Source: CAD feature listing. Evaluate the final solid. Frame: model axes, mm. A direction names the side the tool comes from. Round coordinates to 2 decimals unless told otherwise and drop trailing zeros. Write each loop counter-clockwise with the first axis right and the second up, starting at its lowest first coordinate (ties: lowest second). Pieces come first, ordered by that corner, then holes.
from build123d import *

# Parameters (mm, degrees)
SKETCH1_W                      = 140
SKETCH1_H                      = 44
BASE_FLANGE1_DEPTH             = 1.9
EDGE_FLANGE1_DEPTH             = 140
EDGE_FLANGE1_2_DEPTH           = 140
EDGE_FLANGE2_STRIP_CUT_DEPTH   = 140
EDGE_FLANGE2_STRIP_CUT_2_DEPTH = 140
EDGE_FLANGE2_DEPTH             = 140
EDGE_FLANGE2_BEND_DEPTH        = 140
SKETCH40_R                     = 1
CUT_EXTRUDE1_DEPTH             = 5


# Read off the part's stored shape, not the designer's step: Edge-Flange1
# Sheet-metal steps are written as plain solids
with BuildPart() as part:
    # Sketch1 → Base-Flange1 (new body)
    with BuildSketch(Plane.XY):
        with Locations((70, 22)):
            Rectangle(SKETCH1_W, SKETCH1_H)
    extrude(amount=-BASE_FLANGE1_DEPTH)

    # Edge-Flange1 outline → Edge-Flange1 (cut)
    with BuildSketch(Plane.YZ):
        with BuildLine():
            ThreePointArc((41.266511693, 0), (42.824680557, -0.454164807), (43.894804276, -1.674407041))
            Line((43.894804276, -1.674407041), (44, -1.9))
            Line((44, -1.9), (44, 0))
            Line((44, 0), (41.266511693, 0))
        make_face()
        with BuildLine():
            ThreePointArc((0.105195724, -1.674407041), (1.175319443, -0.454164807), (2.733488307, 0))
            Line((2.733488307, 0), (0, 0))
            Line((0, 0), (0, -1.9))
            Line((0, -1.9), (0.105195724, -1.674407041))
        make_face()
    extrude(amount=EDGE_FLANGE1_DEPTH, mode=Mode.SUBTRACT)

    # Edge-Flange1 2 outline → Edge-Flange1 2 (add)
    with BuildSketch(Plane.YZ):
        with BuildLine():
            Line((44.259494142, -2.456486983), (44, -1.9))
            Line((44, -1.9), (41.266511693, -1.9))
            ThreePointArc((41.266511693, -1.9), (41.803811302, -2.056608554), (42.17281948, -2.477381738))
            Line((42.17281948, -2.477381738), (42.537509347, -3.259461681))
            Line((42.537509347, -3.259461681), (44.259494142, -2.456486983))
        make_face()
        with BuildLine():
            ThreePointArc((1.82718052, -2.477381738), (2.196188698, -2.056608554), (2.733488307, -1.9))
            Line((2.733488307, -1.9), (0, -1.9))
            Line((0, -1.9), (-0.259494142, -2.456486983))
            Line((-0.259494142, -2.456486983), (1.462490653, -3.259461681))
            Line((1.462490653, -3.259461681), (1.82718052, -2.477381738))
        make_face()
    extrude(amount=EDGE_FLANGE1_2_DEPTH)

    # Edge-Flange2 strip (across the edge) → Edge-Flange2 strip cut (cut)
    with BuildSketch(Plane(origin=(140, 44.259494142, -2.456486983), x_dir=(0, 0, 1), z_dir=(-1, 0, 0))):
        Polygon((-8.926147715, 2.065912991), (-0.225592959, -1.991222322), (0.577381738, -0.269237526), (-8.123173017, 3.787897786), align=None)
    extrude(amount=EDGE_FLANGE2_STRIP_CUT_DEPTH, mode=Mode.SUBTRACT)

    # Edge-Flange2 strip 2 (across the edge) → Edge-Flange2 strip cut 2 (cut)
    with BuildSketch(Plane(origin=(0, -0.259494142, -2.456486983), x_dir=(0, 0, 1), z_dir=(1, 0, 0))):
        Polygon((-8.926147715, 2.065912991), (-0.225592959, -1.991222322), (0.577381738, -0.269237526), (-8.123173017, 3.787897786), align=None)
    extrude(amount=EDGE_FLANGE2_STRIP_CUT_2_DEPTH, mode=Mode.SUBTRACT)

    # Edge-Flange2 section (across the edge) → Edge-Flange2 (add)
    with BuildSketch(Plane(origin=(140, 44.259494142, -2.456486983), x_dir=(0, 0, 1), z_dir=(-1, 0, 0))):
        with BuildLine():
            Line((-1.9, 0.637070261), (-1.9, 5))
            Line((-1.9, 5), (0, 5))
            Line((0, 5), (0, 0.637070261))
            ThreePointArc((0, 0.637070261), (0.156608554, 0.099770652), (0.577381738, -0.269237526))
            Line((0.577381738, -0.269237526), (-0.225592959, -1.991222322))
            ThreePointArc((-0.225592959, -1.991222322), (-1.445835193, -0.921098603), (-1.9, 0.637070261))
        make_face()
    extrude(amount=EDGE_FLANGE2_DEPTH)

    # Edge-Flange2 section 2 (across the edge) → Edge-Flange2 bend (add)
    with BuildSketch(Plane(origin=(0, -0.259494142, -2.456486983), x_dir=(0, 0, 1), z_dir=(1, 0, 0))):
        with BuildLine():
            Line((-1.9, 0.637070261), (-1.9, 5))
            Line((-1.9, 5), (0, 5))
            Line((0, 5), (0, 0.637070261))
            ThreePointArc((0, 0.637070261), (0.156608554, 0.099770652), (0.577381738, -0.269237526))
            Line((0.577381738, -0.269237526), (-0.225592959, -1.991222322))
            ThreePointArc((-0.225592959, -1.991222322), (-1.445835193, -0.921098603), (-1.9, 0.637070261))
        make_face()
    extrude(amount=EDGE_FLANGE2_BEND_DEPTH)

    # Sketch40 → Cut-Extrude1 (cut)
    with BuildSketch(Plane.XY):
        with Locations((111, 17.28174)):
            Circle(SKETCH40_R)
        with Locations((43, 17.28174)):
            Circle(SKETCH40_R)
    extrude(amount=-CUT_EXTRUDE1_DEPTH, mode=Mode.SUBTRACT)


solid = part.part
1) Section query A-A on x = 116. Return the cut outline in (y, z).
Taken from the geometry:
outline: (-5.26, -4.36) - (-0.9, -4.36) arc R2.9 ccw to (1.73, -2.68) - (1.83, -2.48) arc R1 cw to (2.73, -1.9) - (41.27, -1.9) arc R1 cw to (42.17, -2.48) - (42.27, -2.68) arc R2.9 ccw to (44.9, -4.36) - (49.26, -4.36) - (49.26, -2.46) - (44.9, -2.46) arc R1 cw to (43.99, -1.88) - (43.89, -1.67) arc R2.9 ccw to (41.27, 0) - (2.73, 0) arc R2.9 ccw to (0.11, -1.67) - (0.01, -1.88) arc R1 cw to (-0.9, -2.46) - (-5.26, -2.46) - close
2) Section query C-C on y = 4.5. Return the cut outline in (x, z), then the cut area to 3 significant figures.
Taken from the geometry:
outline: (0, -1.9) - (140, -1.9) - (140, 0) - (0, 0) - close
area: 266 mm2
3) Section query B-B on z = -0.95. Return the cut outline in (x, y).
Taken from the geometry:
outline: (0, 0.59) - (140, 0.59) - (140, 43.41) - (0, 43.41) - close; hole circle Ø2 at (43, 17.28); hole circle Ø2 at (111, 17.28)
4) Material intervals for line 1 (Z direction, x = 46, y = 18); line 2 (Y direction, x = 111, z = -0.9); line 3 (Y direction, x = 82, z = -2.35), sorted ascending.
Taken from the geometry:
line 1: z = -1.9 to 0
line 2: y = 0.63 to 16.28, 18.28 to 43.37
line 3: y = -0.45 to 1.9, 42.1 to 44.45
5) Reachability of faces 4 (the face through (71, 47, -2.456)), 5 (the face through (69, 22, -1.9)), 6 (the face through (69, -3, -2.456)) from +Z, -Z, +X, -X, +Y, -Y: full face, straight path, thin tool, end or side. Return the list, or none.
Taken from the geometry:
face 4: +Z, +X, -X, +Y
face 5: -Z, +X, -X
face 6: +Z, +X, -X, -Y
6) Pull-direction query (Y, two-part tool) for faces 1 (the face through (70.98, 43.32, -3.89)), 2 (the face through (69.02, 42.805, -0.442)), 3 (the face through (69, -3, -4.356)); classes: released by +Y, released by -Y, zero draft, split by the parting line, or undercut.
Taken from the geometry:
face 1: undercut
face 2: released by +Y
face 3: zero draft
7) Contact query for flat-ended pins moving along their axis: P1, Ø5, axis at x = 45, y = 47.5, coming from the +Z side; P2, Ø1.6, axis at x = 111, y = 17.28, coming from the +Z side; P3, Ø1.5, axis at x = 88.5, z = -1.5, coming from the -Y side; P4, Ø2.5, axis at x = 43, y = 17.28, coming from the -Z side. Output: stop coordinate, or through.
Taken from the geometry:
P1: stops at z = -2.46
P2: passes through
P3: stops at y = -0.29
P4: stops at z = -1.9
